Geometry: see drawing. Coordinates: mm, zero at the bounding-box minimum. Give positions to 0.01 mm unless a question says otherwise; leave off trailing zeros. Write each loop counter-clockwise with the first axis right and the second up, starting at its lowest first coordinate (ties: lowest second). Pieces come first, ordered by that corner, then holes. Notation, with made-up numbers: (52, 77.5) -> (98, 77.5) arc R31 ccw to (98, 105.5) -> close; hole circle Ø6 at (38, 51.25). An arc over 180 degrees is marked (long way). Write item = value, one per line.
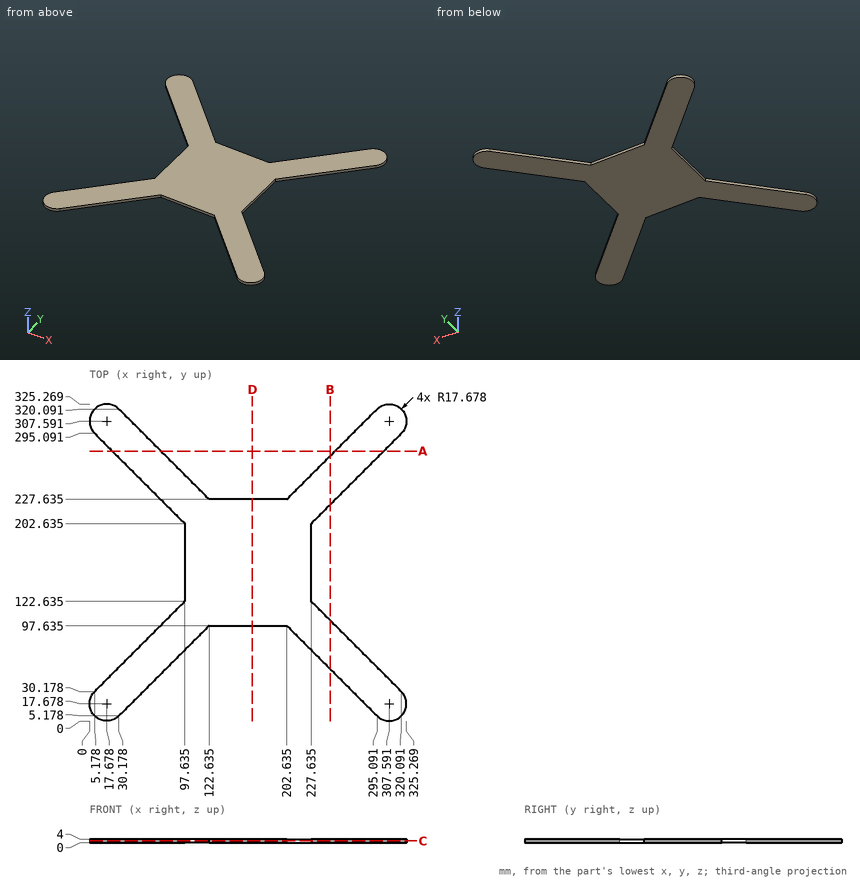
(1) Section query D-D (x = 167). Return loops of the section in (y, z) (1 decimal), plus the area to 3 significant figures.
Values follow:
outline = (97.6, 0) -> (227.6, 0) -> (227.6, 4) -> (97.6, 4) -> close
area = 520 mm2
(2) Section query B-B (x = 247). Return loops of the section in (y, z), plus the area to 3 significant figures.
Values follow:
outline = (53.27, 0) -> (103.27, 0) -> (103.27, 4) -> (53.27, 4) -> close; (222, 0) -> (272, 0) -> (272, 4) -> (222, 4) -> close
area = 400 mm2
(3) First-contact query: pin 1 (2 mm diameter, centred on y = 187.5, z = 3.5, fed in from -X) (1 decimal); pin 2 (1.2 mm diameter, centred on x = 173.5, z = 1.5, fed in from +Y) (1 decimal); pin 3 (1.2 mm diameter, centred on y = 161, z = 2, fed in from +X) (1 decimal). Flat tips, straight axial feed; report the tip coordinate or a pass-through.
Values follow:
pin_1 = 97.6
pin_2 = 227.6
pin_3 = 227.6
(4) Section query C-C (z = 2.15). Return loops of the section in (x, y) (1 decimal), plus the area to 3 significant figures.
Values follow:
outline = (5.2, 30.2) arc R17.7 ccw to (30.2, 5.2) -> (122.6, 97.6) -> (202.6, 97.6) -> (295.1, 5.2) arc R17.7 ccw to (320.1, 30.2) -> (227.6, 122.6) -> (227.6, 202.6) -> (320.1, 295.1) arc R17.7 ccw to (295.1, 320.1) -> (202.6, 227.6) -> (122.6, 227.6) -> (30.2, 320.1) arc R17.7 ccw to (5.2, 295.1) -> (97.6, 202.6) -> (97.6, 122.6) -> close
area = 36,100 mm2
(5) Material intervals for line 1 (X direction, y = 147, z = 3) (1 decimal); line 2 (Y direction, x = 245.5, z = 2.85); line 3 (X direction, y = 26, z = 3.25) (1 decimal), sorted ascending.
Values follow:
line_1 = 97.6 to 227.6
line_2 = 54.77 to 104.77, 220.5 to 270.5
line_3 = 2.1 to 51, 274.3 to 323.2
(6) Section query A-A (y = 277). Return loops of the section in (x, z).
Values follow:
outline = (23.27, 0) -> (73.27, 0) -> (73.27, 4) -> (23.27, 4) -> close; (252, 0) -> (302, 0) -> (302, 4) -> (252, 4) -> close
